```python
from build123d import *

# Parameters (mm, degrees)
F0_R           = 101.6
F1_DEPTH       = 38.1
F2_D           = 13.462
F2_DEPTH       = 50.8
F2_CBORE_D     = 20.32
F2_CBORE_DEPTH = 15.875
F2_TIP         = 4.0443928267
F3_D           = 13.462
F3_DEPTH       = 50.8
F3_CBORE_D     = 20.32
F3_CBORE_DEPTH = 15.875
F3_TIP         = 4.0443928267
F4_ANGLE       = 30
F6_D           = 12.7
F6_DEPTH       = 50.8
F6_CSINK_D     = 14.2875
F6_CSINK_ANGLE = 90
F6_TIP         = 3.8154649308


# Not quite as in the source:
# - a feature names something its author has since deleted; it is built from what else it names


with BuildPart() as f1:
    # F0 (on Front) → F1 (new body)
    with BuildSketch(Plane.XZ):
        Circle(F0_R)
    extrude(amount=-F1_DEPTH)

    # F2
    with Locations(Plane.XZ):
        with Locations((0, 66.675)):
            CounterBoreHole(F2_D / 2, F2_CBORE_D / 2, F2_CBORE_DEPTH, depth=F2_DEPTH)
            with Locations((0, 0, -(F2_DEPTH + F2_TIP / 2))):  # 118° drill point
                Cone(0, F2_D / 2, F2_TIP, mode=Mode.SUBTRACT)

    # F3
    with Locations(Plane.XZ):
        with Locations((-57.7422437973, 33.3375), (-57.7422437973, -33.3375), (0, -66.675), (57.7422437973, -33.3375), (57.7422437973, 33.3375)):
            CounterBoreHole(F3_D / 2, F3_CBORE_D / 2, F3_CBORE_DEPTH, depth=F3_DEPTH)
            with Locations((0, 0, -(F3_DEPTH + F3_TIP / 2))):  # 118° drill point
                Cone(0, F3_D / 2, F3_TIP, mode=Mode.SUBTRACT)


with BuildPart() as f1_1:
    # F4: moved
    add(f1.part.rotate(Axis((0, 0, 0), (0, -1, 0)), F4_ANGLE))


with BuildPart() as f1_2:
    # F5: moved
    add(f1_1.part.moved(Location((-846.1338678, 0, -154.2352516))))

    # F6
    with Locations(Plane.XZ):
        with Locations((-884.2338678, -67.8752516), (-808.0338678, -67.8752516)):
            CounterSinkHole(F6_D / 2, F6_CSINK_D / 2, depth=F6_DEPTH, counter_sink_angle=F6_CSINK_ANGLE)
            with Locations((0, 0, -(F6_DEPTH + F6_TIP / 2))):  # 118° drill point
                Cone(0, F6_D / 2, F6_TIP, mode=Mode.SUBTRACT)


solid = f1_2.part
```
For this review, take the finished solid that the model builds, in its own axes (mm). A direction names the side the tool comes from. Give positions to 0.01 mm unless a question says otherwise; leave off trailing zeros. Write each loop counter-clockwise with the first axis right and the second up, starting at its lowest first coordinate (ties: lowest second). Pieces come first, ordered by that corner, then holes. Notation, with made-up numbers: M -22.75,21 L -0.75,21 A29 ccw -0.75,48 Z; hole C -24.75,86 d2. An arc over 180 degrees is marked long. One line per item, written item: value.
1) For line 1 (X direction, y = 20, z = -154.5); line 2 (Z direction, x = -818, y = 14); line 3 (X direction, y = 29, z = -153), list the stretches that pass through material, from the lowest coordinate up. Write a range as from..to.
Results are:
line 1: x = -947.73..-919.53, -906.08..-786.18, -772.73..-744.53
line 2: z = -251.86..-220.7, -203.25..-105.22, -87.77..-56.61
line 3: x = -947.73..-919.43, -906.19..-786.08, -772.84..-744.54
2) For P1, Ø16.5, axis at x = -879.5, z = -211, coming from the -Y side (3 decimals); P2, Ø4, axis at x = -894, y = 10.5, coming from the -Z side; P3, Ø23.5, axis at x = -779.46, z = -154.24, coming from the +Y side; P4, Ø8, axis at y = 14, z = -129, coming from the +X side, all flat-tipped, find the tip position at first contact; note any pin that passes through.
Results are:
P1: stops at y = 15.875
P2: stops at z = -244.89
P3: stops at y = 38.1
P4: stops at x = -746.78
3) Take a section at B-B, the plane y = 27.5. Count the separate pieces of the cut face and the enclosed holes in it, then the cut area to 3 significant figures.
Results are:
separate pieces: 1
enclosed holes: 8
area: 31,300 mm²
4) The part is to be moulded in two halves that separate along Z. For faces 1 (the cylindrical face through (-945.318, 18.783, -132.21)), 2 (the cylindrical face through (-869.4, 7.83, -210.65)), 3 (the flat face through (-848, 38.1, -154)), say which applies: +Z half, -Z half, draft (parallel to the pull), parting line (faces both ways), or undercut.
Results are:
face 1: parting line
face 2: undercut
face 3: draft
5) Take a section at A-A, the plane z = -151.5. Write out the cut boundary in (x, y) (3 decimals).
Results are:
outline: M -947.697,0 L -922.594,0 L -922.594,15.875 L -918.959,15.875 L -918.959,38.1 L -947.697,38.1 Z; M -906.659,15.875 L -903.024,15.875 L -903.024,0 L -789.244,0 L -789.244,15.875 L -785.609,15.875 L -785.609,38.1 L -906.659,38.1 Z; M -773.309,15.875 L -769.674,15.875 L -769.674,0 L -744.571,0 L -744.571,38.1 L -773.309,38.1 Z
6) For faces 4 (the cylindrical face through (-808.247, 27.143, -101.454)), 5 (the flat face through (-772.7, 15.875, -152.8)), list the 3-axis set-ups (+Z, -Z, +X, -X, +Y, -Y) from which the entire face can be reached by the end or side of a thin tool; tool diameter is ignored.
Results are:
face 4: +Y, -Y
face 5: -Y
7) Take a section at D-D, the plane z = -198.5. Write out the cut boundary in (x, y).
Results are:
outline: M -937.58,0 L -754.68,0 L -754.68,38.1 L -937.58,38.1 Z
